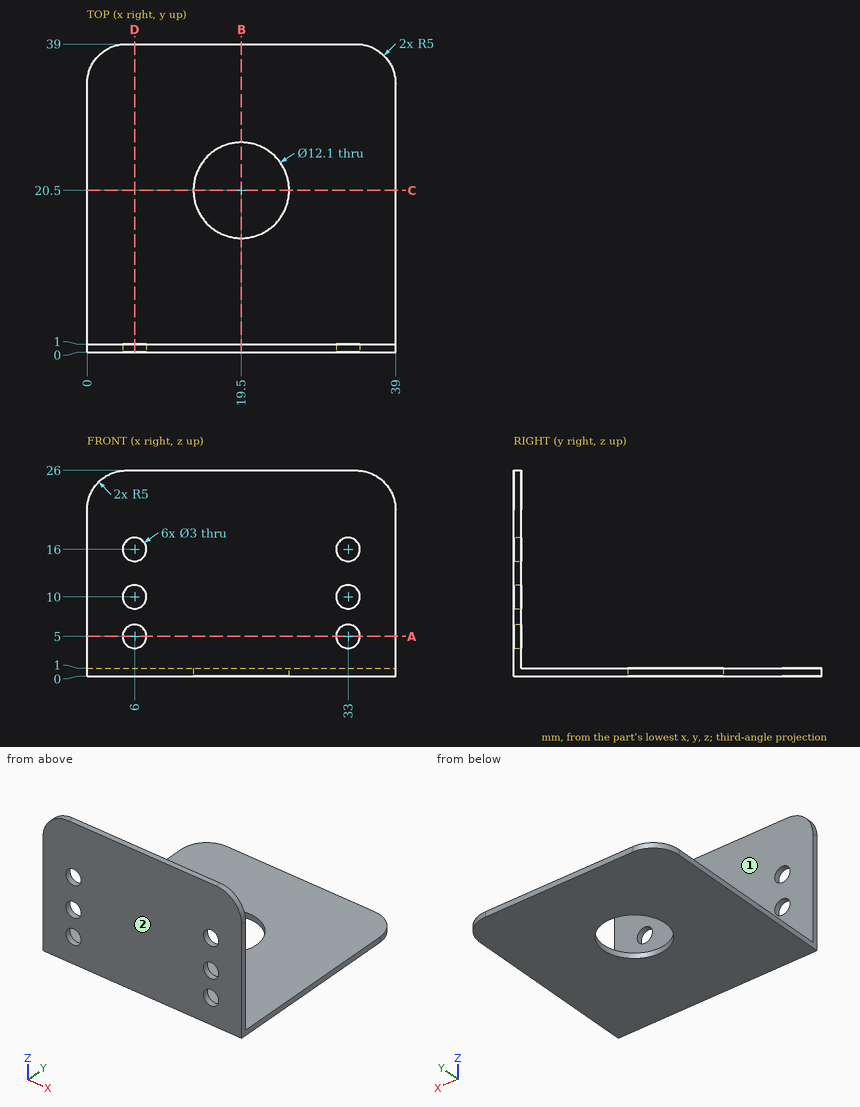
Input: dimensioned drawing with shaded views. Units: mm. Origin: part minimum x, y, z. A direction names the side the tool comes from. Coordinates: 2 decimals unless noted, no trailing zeros. Loops run counter-clockwise (first coordinate to the right, second up) from the corner with the lowest first, then second, coordinate; pieces in that order, holes last. Notation, with made-up numbers: M 4.5,12 L 59.5,12 A10 cw 59.5,26 Z; hole C 43,20.5 d9. An arc over 180 degrees is marked long. One line per item, written item: value. Start each with the question number.
1) Cut plane B-B (x = 19.5). Return loops of the section in (y, z).
2) Material intervals for L1, parallel to X at y = 0.75, z = 16; L2, parallel to Y at x = 19.5, z = 0.8; L3, parallel to Y at x = 35, z = 2.75, sorted ascending. Write a range as from..to.
3) Pin query (flat end, axial travel): P1, Ø12, axis at x = 32.5, y = 24.5, coming from the +Z side; P2, Ø2.5, axis at x = 6, z = 5, coming from the -Y side; P3, Ø3.5, axis at x = 6, z = 16, coming from the +Y side. Return the tip coordinate at first contact, or that it passes through.
4) Cut plane C-C (y = 20.5). Return loops of the section in (x, z).
5) Cut plane D-D (x = 6). Return loops of the section in (y, z), then the cut area to 3 significant figures.
6) Reachability of the marked faces 1 and 2 from +Z, -Z, +X, -X, +Y, -Y: full face, straight path, thin tool, end or side. Return the list, or none.
7) Cut plane A-A (z = 5). Return loops of the section in (x, y).
Evaluation:
1. outline: M 0,0 L 14.45,0 L 14.45,1 L 1,1 L 1,26 L 0,26 Z; M 26.55,0 L 39,0 L 39,1 L 26.55,1 Z
2. L1: 0..4.5, 7.5..31.5, 34.5..39
2. L2: 0..14.45, 26.55..39
2. L3: 0..1
3. P1: z = 1
3. P2: through
3. P3: y = 1
4. outline: M 0,0 L 13.45,0 L 13.45,1 L 0,1 Z; M 25.55,0 L 39,0 L 39,1 L 25.55,1 Z
5. outline: M 0,0 L 39,0 L 39,1 L 1,1 L 1,3.5 L 0,3.5 Z; M 0,6.5 L 1,6.5 L 1,8.5 L 0,8.5 Z; M 0,11.5 L 1,11.5 L 1,14.5 L 0,14.5 Z; M 0,17.5 L 1,17.5 L 1,26 L 0,26 Z
5. area: 55.0 mm^2
6. face 1: +Z, +X, -X, +Y
6. face 2: +Z, -Z, +X, -X, -Y
7. outline: M 0,0 L 4.5,0 L 4.5,1 L 0,1 Z; M 7.5,0 L 31.5,0 L 31.5,1 L 7.5,1 Z; M 34.5,0 L 39,0 L 39,1 L 34.5,1 Z
